from build123d import *

# Parameters (mm, degrees)
ESQUISSE1_R             = 11.55
ESQUISSE1_R_2           = 3.025
BOSS_EXTRU_1_DEPTH      = 6.95
ESQUISSE2_R             = 13.660407535
ESQUISSE2_R_2           = 7.85
ENL_V_MAT_EXTRU_1_DEPTH = 5.15
ESQUISSE4_R             = 4.7
ESQUISSE4_R_2           = 3.025
BOSS_EXTRU_2_DEPTH      = 5.5
ESQUISSE5_R             = 2
ENL_V_MAT_EXTRU_3_DEPTH = 21.537952673


with BuildPart() as part:
    # Esquisse1 → Boss.-Extru.1 (new, symmetric)
    with BuildSketch(Plane.XY):
        Circle(ESQUISSE1_R)
        Circle(ESQUISSE1_R_2, mode=Mode.SUBTRACT)
    extrude(amount=BOSS_EXTRU_1_DEPTH, both=True)

    # Esquisse2 → Enlèv. mat.-Extru.1 (cut, symmetric)
    with BuildSketch(Plane.XY):
        Circle(ESQUISSE2_R)
        Circle(ESQUISSE2_R_2, mode=Mode.SUBTRACT)
    extrude(amount=ENL_V_MAT_EXTRU_1_DEPTH, both=True, mode=Mode.SUBTRACT)

    # Esquisse4 → Boss.-Extru.2 (add)
    with BuildSketch(Plane.XY.offset(6.95)):
        Circle(ESQUISSE4_R)
        Circle(ESQUISSE4_R_2, mode=Mode.SUBTRACT)
    extrude(amount=BOSS_EXTRU_2_DEPTH)

    # Esquisse5 → Enlèv. mat.-Extru.3 (cut, through all)
    with BuildSketch(Plane(origin=(0, 0, 0), x_dir=(1, 0, 0), z_dir=(0, 1, 0))):
        with Locations(Location((0, -9.7, 0), (0, 0, 90))):
            Circle(ESQUISSE5_R)
    extrude(amount=ENL_V_MAT_EXTRU_3_DEPTH, mode=Mode.SUBTRACT)


solid = part.part
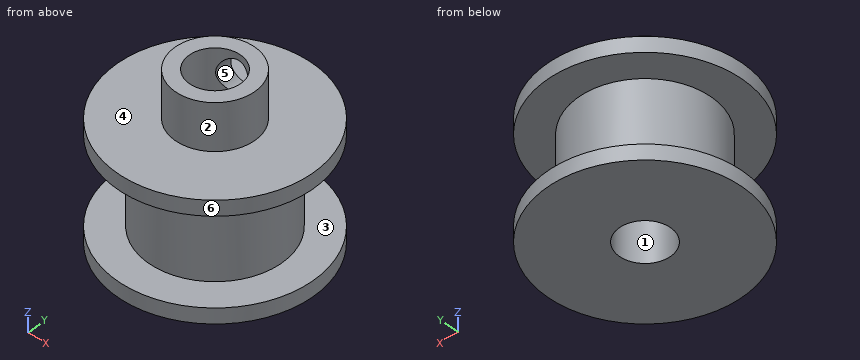
Geometry: final body of the model. Coordinates: model frame, mm. Face numbers are marked on the shaded views. A direction names the side the tool comes from. Coordinates: 2 decimals unless noted, no trailing zeros. Loops run counter-clockwise (first coordinate to the right, second up) from the corner with the lowest first, then second, coordinate; pieces in that order, holes last. Notation, with made-up numbers: (-25, -11) - (-10, -11) arc R6 ccw to (-10, -1) - close; hole circle Ø7 at (5, 35). An arc over 180 degrees is marked (long way). One line per question, with ' | ' between items. Start each with the question number.
(1) Cut plane A-A on y = 8.5. Output: boundary loops of the cut face in (x, z).
(2) Reachability of the marked faces 1, 2 and 3 from +Z, -Z, +X, -X, +Y, -Y: full face, straight path, thin tool, end or side. Return the list, or none.
(3) Ray query, L1, parallel to Z at x = -8, y = -6.75; L2, parallel to Z at x = 0.5, y = -6.5; L3, parallel to Y at x = 0, z = -1 (3 decimals). Return the intervals inside material, ascending. Write a range as from..to.
(4) Draft query along Z for the marked faces 4, 5 and 6. Return one class per face: +Z half, -Z half, draft (parallel to the pull), parting line (faces both ways), or undercut.
(5) First-contact query: pin 1 (10 mm diameter, centred on x = -5.5, z = -2, fed in from -Y); pin 2 (1.5 mm diameter, centred on x = -3, z = 9.5, fed in from -Y); pin 3 (3 mm diameter, centred on y = -7, z = 5, fed in from -X). Flat tips, straight axial feed; report the tip coordinate or a pass-through.
(6) Cut plane D-D on z = -0.5. Output: boundary loops of the cut face in (x, y) (3 decimals), and give its area (3 significant figures).
(7) Cut plane B-B on x = 0. Output: boundary loops of the cut face in (y, z) (3 decimals).
(8) Cut plane C-C on x = -9. Output: boundary loops of the cut face in (y, z).
Here are the results:
1) outline: (-7.82, -6.95) - (7.82, -6.95) - (7.82, -5.15) - (-7.82, -5.15) - close; (-7.82, 5.15) - (7.82, 5.15) - (7.82, 6.95) - (-7.82, 6.95) - close
2) face 1: +Z, -Z | face 2: +Z | face 3: none
3) L1: -6.95..-5.15, 5.15..6.95 | L2: -6.95..6.95 | L3: -7.85..-3.025, 3.025..7.85
4) face 4: +Z half | face 5: undercut | face 6: draft
5) pin 1: y = -11.44 | pin 2: y = -4.13 | pin 3: x = -10.15
6) outline: circle Ø15.7 at (0, 0); hole circle Ø6.05 at (0, 0) | area: 165 mm²
7) outline: (-11.55, -6.95) - (-3.025, -6.95) - (-3.025, 12.45) - (-4.7, 12.45) - (-4.7, 6.95) - (-11.55, 6.95) - (-11.55, 5.15) - (-7.85, 5.15) - (-7.85, -5.15) - (-11.55, -5.15) - close; (3.025, -6.95) - (11.55, -6.95) - (11.55, -5.15) - (7.85, -5.15) - (7.85, 5.15) - (11.55, 5.15) - (11.55, 6.95) - (4.7, 6.95) - (4.7, 7.7) - (3.025, 7.7) - close; (3.025, 11.7) - (4.7, 11.7) - (4.7, 12.45) - (3.025, 12.45) - close
8) outline: (-7.24, -6.95) - (7.24, -6.95) - (7.24, -5.15) - (-7.24, -5.15) - close; (-7.24, 5.15) - (7.24, 5.15) - (7.24, 6.95) - (-7.24, 6.95) - close
